Design review of the part built by this model. Coordinates are the model's own, in mm. A direction names the side the tool comes from. Coordinates: 2 decimals unless noted, no trailing zeros. Write each loop counter-clockwise with the first axis right and the second up, starting at its lowest first coordinate (ties: lowest second). Pieces come first, ordered by that corner, then holes. Notation, with made-up numbers: (-6.5, 58.25) - (37.5, 58.25) arc R21 ccw to (37.5, 71.25) - close; hole circle Ø11 at (61, 43). An arc over 180 degrees is marked (long way). One line per item, written item: value.
from build123d import *

# Parameters (mm, degrees)
F1_DEPTH = 51.5
F2_W     = 13
F2_H     = 22.75
F3_DEPTH = 13
F4_W     = 13
F4_H     = 3
F5_DEPTH = 5


with BuildPart() as f1:
    # F0 (on Front) → F1 (new body)
    with BuildSketch(Plane.XZ):
        Polygon((5, 0), (29.50686, 0), (10.25, 26.798756), (-10.25, 26.798756), (-29.50686, 0), (-5, 0), (-5, 8.67), (5, 8.67), align=None)
    extrude(amount=F1_DEPTH)

    # F2 (on face) → F3 (cut)
    with BuildSketch(Plane.XZ.offset(51.5)):
        with Locations((0, 15.423756)):
            Rectangle(F2_W, F2_H)
    extrude(amount=-F3_DEPTH, mode=Mode.SUBTRACT)

    # F4 (on face) → F5 (cut)
    with BuildSketch(Plane.XZ.offset(38.5)):
        with Locations((-0.192779, 23.298756)):
            Rectangle(F4_W, F4_H)
    extrude(amount=-F5_DEPTH, mode=Mode.SUBTRACT)


solid = f1.part
1. Wall thickness on line 1 along X through (y, z) = (-47.5, 2.75); line 2 along X through (y, z) = (-28.5, 5.5); line 3 along Y through (x, z) = (-6, 24.25): over which ranges is each line inside the solid? List them lowest first.
Answer block:
line 1: x = -27.53 to -5, 5 to 27.53
line 2: x = -25.55 to -5, 5 to 25.55
line 3: y = -33.5 to 0
2. Consider section B-B, the plane x = 2. Write out the cut boundary in (y, z).
Answer block:
outline: (-38.5, 8.67) - (0, 8.67) - (0, 26.8) - (-38.5, 26.8) - (-38.5, 24.8) - (-33.5, 24.8) - (-33.5, 21.8) - (-38.5, 21.8) - close
3. For faces 5 (the face through (6.307, -36, 23)), 6 (the face through (-5, -25, 4)), 7 (the face through (-6, -45, 4.049)), list the 3-axis set-ups (+Z, -Z, +X, -X, +Y, -Y) from which the entire face can be reached by the end or side of a thin tool; tool diameter is ignored.
Answer block:
face 5: -Y
face 6: -Z, +Y, -Y
face 7: +Z, -Y
4. Consider section A-A, the plane y = -46.5. Write out the cut boundary in (x, z).
Answer block:
outline: (-29.51, 0) - (-5, 0) - (-5, 4.05) - (-6.5, 4.05) - (-6.5, 26.8) - (-10.25, 26.8) - close; (5, 0) - (29.51, 0) - (10.25, 26.8) - (6.5, 26.8) - (6.5, 4.05) - (5, 4.05) - close
5. Mouldability with a two-part tool opening along X and no side actions: class faces 1 (the face through (-19.74, -25.39, 13.59)), 2 (the face through (0, -36, 24.799)), 3 (the face through (20.013, -25.39, 13.212)), 4 (the face through (17, -25, 0)) as released by +X, released by -X, zero draft, split by the parting line, or undercut.
Answer block:
face 1: released by -X
face 2: undercut
face 3: released by +X
face 4: zero draft
6. Consider section C-C, the plane z = 7.25. Write out the cut boundary in (x, y).
Answer block:
outline: (-24.3, -51.5) - (-6.5, -51.5) - (-6.5, -38.5) - (-5, -38.5) - (-5, 0) - (-24.3, 0) - close; (5, -38.5) - (6.5, -38.5) - (6.5, -51.5) - (24.3, -51.5) - (24.3, 0) - (5, 0) - close
7. Insertion check: pin 1 Ø4 at (y, z) = (-26, 4.5) entering from -X; pin 2 Ø0.9 at (y, z) = (-37, 23) entering from +X; pin 3 Ø0.8 at (x, y) = (6, -46.5) entering from +Z. Each pin has a flat end and moves straight along its axis. Give the tip position at first contact, or say it passes through.
Answer block:
pin 1: stops at x = -27.71
pin 2: stops at x = 13.3
pin 3: stops at z = 4.05
8. Consider section D-D, the plane y = -13. Write out the cut boundary in (x, z), then the cut area to 3 significant figures.
Answer block:
outline: (-29.51, 0) - (-5, 0) - (-5, 8.67) - (5, 8.67) - (5, 0) - (29.51, 0) - (10.25, 26.8) - (-10.25, 26.8) - close
area: 979 mm^2
